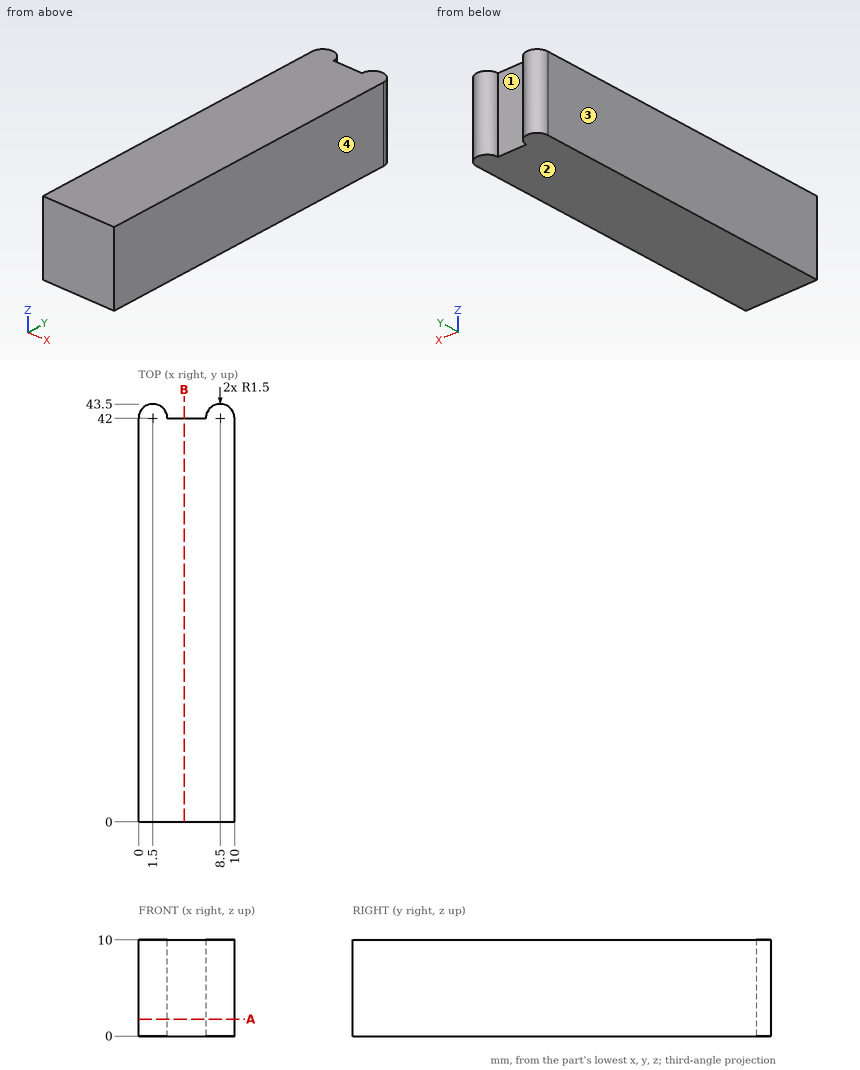
Could you check a few things on this drawing? It's one solid part, dimensions in mm from its lowest x, y, z. Coordinates: 2 decimals unless noted, no trailing zeros. Loops run counter-clockwise (first coordinate to the right, second up) from the corner with the lowest first, then second, coordinate; pieces in that order, holes last. Notation, with made-up numbers: (63, 2) - (67, 2) arc R15 cw to (67, 22) - close; hole circle Ø8 at (42.25, 36). An arc over 180 degrees is marked (long way). Answer as a JSON object with one key per item and string values. Group by question number.
Item 1: For pin 1 (4.5 mm diameter, centred on x = 5.5, z = 7, fed in from +Y), with a flat end and sliding along its axis, tell me the tip position at first contact or that it passes through.
Item 2: If I drill on L1, parallel to Y at x = 3.75, z = 3.25; L2, parallel to Y at x = 8, z = 5.75, over which ranges is the centre line in solid material (lowest first)? Write a range as from..to.
Item 3: If we section it at B-B (x = 4.75): List the corners of the cut face in (y, z) for me.
Item 4: If we mould it in two halves opening along X, with no side actions, what happens to the marked faces 1, 2, 3 and 4? For each: released by +X, released by -X, zero draft, split by the parting line, or undercut.
Item 5: If we section it at A-A (z = 1.75): List the corners of the cut face in (x, y) for me.
Returned:
{
 "1": {"pin 1": "stops at y = 43.3"},
 "2": {"L1": "y = 0..42", "L2": "y = 0..43.41"},
 "3": {"outline": "(0, 0) - (42, 0) - (42, 10) - (0, 10) - close"},
 "4": {"face 1": "undercut", "face 2": "zero draft", "face 3": "released by -X", "face 4": "released by +X"},
 "5": {"outline": "(0, 0) - (10, 0) - (10, 42) arc R1.5 ccw to (7, 42) - (3, 42) arc R1.5 ccw to (0, 42) - close"}
}
